Work out the finished part from the listing and answer in its coordinate system (mm). Face numbers are marked on the shaded views. Round coordinates to 2 decimals unless told otherwise and drop trailing zeros. Write each loop counter-clockwise with the first axis right and the second up, starting at its lowest first coordinate (ties: lowest second). Pieces come first, ordered by that corner, then holes.
1. Find section B-B (y = -6.5). Write down the section's boundary in (x, z).
2. Find section C-C (z = 8.5). Write down the section's boundary in (x, y), and give its area (3 significant figures).
3. Flat-ended cylindrical pins translate along their axes: pin 1 Ø6 at (x, z) = (4.5, 6) entering from +Y; pin 2 Ø5 at (x, z) = (4, 4) entering from -Y; pin 3 Ø10 at (x, y) = (-6, 16) entering from +Z; pin 4 Ø1.5 at (y, z) = (-31.5, 8) entering from +X. Find the tip coordinate at first contact, or state that the pin passes through.
4. Determine the mould class of the marked faces 1, 2, 3 and 4 for opening direction X: pulls with the +X half, pulls with the -X half, needs draft (parallel to the pull), parting line crosses it, or undercut.
5. Find section A-A (x = 0). Write down the section's boundary in (y, z), and give its area (3 significant figures).
6. Straight lines are drawn through the part: probe 1 along Y at (x, z) = (0, 6); probe 2 along X at (y, z) = (0.5, 0.5); probe 3 along Y at (x, z) = (21.5, 3.5). For each, find the intervals that lie inside material, in ascending order.
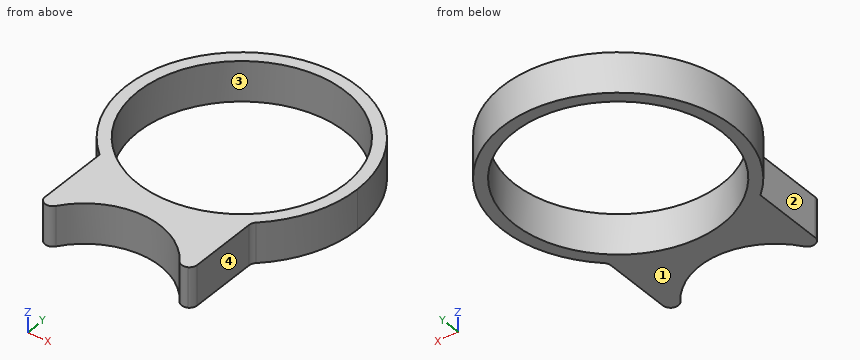
```python
from build123d import *

# Parameters (mm, degrees)
F0_R        = 26
F1_DEPTH    = 10
F2_T1_DEPTH = 10
F2_T3_DEPTH = 15.7735026919
F2_T5_DEPTH = 19.5643999635


# Not quite as in the source:
# - a fillet or chamfer that OpenCascade refuses, or shapes differently, is made with other operations: its cross-section is extruded or revolved along the edge and cut away or added


with BuildPart() as f1:
    # F0 (on Top) → F1 (new body)
    with BuildSketch(Plane.XY):
        with BuildLine():
            ThreePointArc((19.0958601534, -21.8254009127), (26.4081421578, -11.9837401413), (29, 0))
            ThreePointArc((29, 0), (-11.9837401413, 26.4081421578), (-19.0958601534, -21.8254009127))
            ThreePointArc((-19.0958601534, -21.8254009127), (0, -29), (19.0958601534, -21.8254009127))
        make_face()
        Circle(F0_R, mode=Mode.SUBTRACT)
        with BuildLine():
            ThreePointArc((19.0958601534, -21.8254009127), (0, -29), (-19.0958601534, -21.8254009127))
            Line((-19.0958601534, -21.8254009127), (-19.0958601534, -40.975))
            ThreePointArc((-19.0958601534, -40.975), (0, -29.8996567452), (19.0958601534, -40.975))
            Line((19.0958601534, -40.975), (19.0958601534, -21.8254009127))
        make_face()
        with BuildLine():
            ThreePointArc((19.0958601534, -40.975), (0, -29.8996567452), (-19.0958601534, -40.975))
            Line((-19.0958601534, -40.975), (-16.4977839421, -42.475))
            ThreePointArc((-16.4977839421, -42.475), (0, -32.8996021136), (16.4977839421, -42.475))
            Line((16.4977839421, -42.475), (19.0958601534, -40.975))
        make_face()
    extrude(amount=F1_DEPTH)

    # F2: fillet of radius 2 on 5 edges, made by hand

    # F2_s2 → F2_t1 (join)
    with BuildSketch(Plane.XY):
        with BuildLine():
            ThreePointArc((19.7348369177, -21.2493814458), (19.2625507863, -21.9154958064), (19.0958601534, -22.7148560283))
            Line((19.0958601534, -22.7148560283), (19.0958601534, -21.8254009127))
            ThreePointArc((19.0958601534, -21.8254009127), (19.4174846045, -21.5397607144), (19.7348369177, -21.2493814458))
        make_face()
    extrude(amount=F2_T1_DEPTH)

    # F2_s4 → F2_t3 (cut)
    with BuildSketch(Plane.XY.offset(-2.8867513459)):
        with BuildLine():
            ThreePointArc((-19.0958601534, -39.8202994616), (-18.827910961, -40.8202994616), (-18.0958601534, -41.5523502692))
            Line((-18.0958601534, -41.5523502692), (-19.0958601534, -40.975))
            Line((-19.0958601534, -40.975), (-19.0958601534, -39.8202994616))
        make_face()
        with BuildLine():
            ThreePointArc((18.0958601534, -41.5523502692), (18.827910961, -40.8202994616), (19.0958601534, -39.8202994616))
            Line((19.0958601534, -39.8202994616), (19.0958601534, -40.975))
            Line((19.0958601534, -40.975), (18.0958601534, -41.5523502692))
        make_face()
    extrude(amount=F2_T3_DEPTH, mode=Mode.SUBTRACT)

    # F2_s6 → F2_t5 (cut)
    with BuildSketch(Plane.XY.offset(-4.7821999818)):
        with BuildLine():
            ThreePointArc((-18.1543866102, -41.5185600036), (-16.7253721793, -41.7399540041), (-15.5206355044, -40.940137093))
            ThreePointArc((-15.5206355044, -40.940137093), (-16.0275933003, -41.6958649061), (-16.4977839421, -42.475))
            Line((-16.4977839421, -42.475), (-18.1543866102, -41.5185600036))
        make_face()
        with BuildLine():
            ThreePointArc((15.5206355044, -40.940137093), (16.7253721793, -41.7399540041), (18.1543866102, -41.5185600036))
            Line((18.1543866102, -41.5185600036), (16.4977839421, -42.475))
            ThreePointArc((16.4977839421, -42.475), (16.0275933003, -41.6958649061), (15.5206355044, -40.940137093))
        make_face()
    extrude(amount=F2_T5_DEPTH, mode=Mode.SUBTRACT)


solid = f1.part
```
Worked answers:
1. outline: (-28.26, 0) - (-25.17, 0) - (-25.17, 10) - (-28.26, 10) - close; (25.17, 0) - (28.26, 0) - (28.26, 10) - (25.17, 10) - close
2. outline: (-19.1, -39.82) arc R2 ccw to (-18.12, -41.54) arc R2 ccw to (-15.52, -40.94) arc R19 cw to (15.52, -40.94) arc R2 ccw to (18.12, -41.54) arc R2 ccw to (19.1, -39.82) - (19.1, -22.71) arc R2 cw to (19.73, -21.25) arc R29 ccw (long way) to (-19.1, -21.83) - close; hole circle Ø52 at (0, 0)
2. area: 889 mm2
3. pin 1: stops at y = 28.96
3. pin 2: stops at y = -34.05
3. pin 3: passes through
3. pin 4: stops at x = 19.1
4. face 1: needs draft
4. face 2: pulls with the -X half
4. face 3: undercut
4. face 4: pulls with the +X half
5. outline: (-32.9, 0) - (-26, 0) - (-26, 10) - (-32.9, 10) - close; (26, 0) - (29, 0) - (29, 10) - (26, 10) - close
5. area: 99.0 mm2
6. probe 1: y = -32.9 to -26, 26 to 29
6. probe 2: x = -29 to -26, 26 to 29
6. probe 3: y = -19.46 to -14.62, 14.62 to 19.46
